CAD build for the part. Positions are in the model's coordinates, mm. A direction names the side the tool comes from. Give positions to 0.01 mm unless a question says otherwise; leave off trailing zeros. Write each loop counter-clockwise with the first axis right and the second up, starting at its lowest first coordinate (ties: lowest second). Pieces come first, ordered by that corner, then holes. Notation, with made-up numbers: M 45.5,62.5 L 50.5,62.5 A27 ccw 50.5,87.5 Z; hole C -9,-27 d5. An arc over 180 degrees is marked long. One line per question, with ' | ' between items. Start each with the question number.
1. Cut at B-B, the plane x = -34. Write the cut outline in (y, z), then the cut area to 4 significant figures.
2. Cut at A-A, the plane y = -2.2. Count the separate pieces of the cut face and the enclosed holes in it, then the cut area to 3 significant figures.
3. Cut at D-D, the plane x = -18. Write the cut outline in (y, z).
4. Pull direction Z, two halves, no side cores. Call faces 1 (the face through (-36.5, 0, -7.5)), 2 (the face through (0, 0, -12)), 3 (the face through (-20.365, 0.036, -0.987)): released by +Z, released by -Z, zero draft, split by the parting line, or undercut.
5. Flat gauge pins, fed straight in: pin 1 (4.5 mm diameter, centred on x = -4.5, z = -3.5, fed in from +Y); pin 2 (2.5 mm diameter, centred on x = -4, z = -3.5, fed in from +Y); pin 3 (0.8 mm diameter, centred on x = -34, z = 0.5, fed in from -Y); pin 4 (0.8 mm diameter, centred on x = -4.5, y = 1.5, fed in from +Z). Where does each tip first touch, or does it go through?
6. Cut at C-C, the plane z = -22.25. Write the cut outline in (x, y).
7. Wall check: L1, parallel to Z at x = -4, y = -1.55; L2, parallel to X at y = -0.65, z = -3.25; L3, parallel to Z at x = -5, y = -2.1. Give the ranges that are in metal, low to high.
8. Which spindle directions (+Z, -Z, +X, -X, +Y, -Y) get a long thin tool onto all of the face, cutting with end or side? Do faces 4 (the face through (-3, 0.1, -23)), 5 (the face through (-17, 0, -2)), 6 (the face through (-9.5, -2.1, 2.5)), 7 (the face through (-36.5, 1.9, -0.5)), 8 (the face through (-36.5, -1.9, -0.5)). Say none if no direction does.
```python
from build123d import *

# Parameters (mm, degrees)
BOSS_EXTRUDE1_DEPTH = 2.6
BOSS_EXTRUDE2_DEPTH = 4
BOSS_EXTRUDE3_DEPTH = 4
SKETCH4_W           = 3
SKETCH4_H           = 5.2
BOSS_EXTRUDE4_DEPTH = 8
BOSS_EXTRUDE5_DEPTH = 2.6
SKETCH6_R           = 1.6
CUT_EXTRUDE1_DEPTH  = 6.2
CUT_EXTRUDE2_DEPTH  = 2.5
CHAMFER1_SIZE       = 1


with BuildPart() as part:
    # Sketch1 → Boss-Extrude1 (new body, symmetric)
    with BuildSketch(Plane(origin=(0, 0, 0), x_dir=(1, 0, 0), z_dir=(0, 1, 0))):
        Polygon((0, 0), (0, 25), (-8, 25), (-8, 8), (-37, 8), (-37, 0), (-33, 0), (-33, 2), (-25, 2), (-25, 0), (-21, 0), (-21, 2), (-13, 2), (-13, 0), align=None)
    extrude(amount=BOSS_EXTRUDE1_DEPTH, both=True)

    # Sketch2 → Boss-Extrude2 (add)
    with BuildSketch(Plane.ZY.offset(13)):
        Polygon((1.5, -1.25), (1.5, -2.6), (4.5, -2.6), (4.5, 2.6), (1.5, 2.6), (1.5, 1.25), (0, 1.25), (0, -1.25), align=None)
    boss_extrude2 = extrude(amount=-BOSS_EXTRUDE2_DEPTH)

    # Sketch3 → Boss-Extrude3 (add)
    with BuildSketch(Plane.ZY.offset(25)):
        Polygon((0, 1.25), (0, -1.25), (1.5, -1.25), (1.5, -2.6), (4.5, -2.6), (4.5, 2.6), (1.5, 2.6), (1.5, 1.25), align=None)
    extrude(amount=-BOSS_EXTRUDE3_DEPTH)

    # Sketch4 → Boss-Extrude4 (add)
    with BuildSketch(Plane.ZY.offset(13)):
        with Locations((3, 0)):
            Rectangle(SKETCH4_W, SKETCH4_H)
    boss_extrude4 = extrude(amount=BOSS_EXTRUDE4_DEPTH)

    # Sketch5 → Boss-Extrude5 (add, symmetric)
    with BuildSketch(Plane(origin=(0, 0, 0), x_dir=(1, 0, 0), z_dir=(0, 1, 0))):
        with BuildLine():
            Line((-13, 1), (-13, 2))
            Line((-13, 2), (-13.535898385, 2))
            ThreePointArc((-13.535898385, 2), (-16.36772326, 0.050287843), (-19.666666667, 1.01857603))
            ThreePointArc((-19.666666667, 1.01857603), (-20.372677996, 0.979231367), (-20.333333333, 0.273220038))
            ThreePointArc((-20.333333333, 0.273220038), (-16.506884, -0.975624243), (-13, 1))
        make_face()
    boss_extrude5 = extrude(amount=BOSS_EXTRUDE5_DEPTH, both=True)

    # Mirror1: Boss-Extrude2, Boss-Extrude4, Boss-Extrude5 across plane
    add(boss_extrude2.mirror(Plane.ZY.offset(23)))
    add(boss_extrude4.mirror(Plane.ZY.offset(23)))
    add(boss_extrude5.mirror(Plane.ZY.offset(23)))

    # Sketch6 → Cut-Extrude1 (cut, through all)
    with BuildSketch(Plane(origin=(0, 2.6, 0), x_dir=(1, 0, 0), z_dir=(0, 1, 0))):
        with Locations((-4, 21.5)):
            Circle(SKETCH6_R)
        with Locations((-4, 3.5)):
            Circle(SKETCH6_R)
    extrude(amount=-CUT_EXTRUDE1_DEPTH, mode=Mode.SUBTRACT)

    # Sketch7 → Cut-Extrude2 (cut)
    with BuildSketch(Plane(origin=(0, 2.6, 0), x_dir=(1, 0, 0), z_dir=(0, 1, 0))):
        Polygon((-0.824573519, 3.5), (-2.41228676, 6.25), (-5.58771324, 6.25), (-7.175426481, 3.5), (-5.58771324, 0.75), (-2.41228676, 0.75), align=None)
        Polygon((-0.824573519, 21.5), (-2.41228676, 24.25), (-5.58771324, 24.25), (-7.175426481, 21.5), (-5.58771324, 18.75), (-2.41228676, 18.75), align=None)
    extrude(amount=-CUT_EXTRUDE2_DEPTH, mode=Mode.SUBTRACT)

    # Chamfer1
    chamfer1_edges = [part.edges().sort_by_distance(p)[0] for p in [
        (-9, 0, 4.5),
        (-9, -2.6, 3),
        (-23, -2.6, 4.5),
        (-9, 2.6, 3),
        (-23, 2.6, 4.5),
        (-37, -2.6, 3),
        (-37, 2.6, 3),
        (-37, 0, 4.5),
        (-37, 1.925, 0),
        (-37, -1.925, 0),
        (-37, 0, -8),
        (-8, 0, -8),
        (0, 0, 0),
        (0, 0, -25),
        (-8, 0, -25),
    ]]
    chamfer(chamfer1_edges, length=CHAMFER1_SIZE)


solid = part.part
```
Here are the results:
1) outline: M -2.6,-8 L 2.6,-8 L 2.6,0 L 1.25,0 L 1.25,1.5 L 2.6,1.5 L 2.6,3.5 L 1.6,4.5 L -1.6,4.5 L -2.6,3.5 L -2.6,1.5 L -1.25,1.5 L -1.25,0 L -2.6,0 Z | area: 59.95 mm^2
2) separate pieces: 2 | enclosed holes: 2 | area: 463 mm^2
3) outline: M -2.6,-8 L 2.6,-8 L 2.6,-2 L -2.6,-2 Z; M -2.6,-0.13 L 2.6,-0.13 L 2.6,0.9 L -2.6,0.9 Z; M -2.6,1.5 L 2.6,1.5 L 2.6,3.5 L 1.6,4.5 L -1.6,4.5 L -2.6,3.5 Z
4) face 1: released by -Z | face 2: zero draft | face 3: undercut
5) pin 1: y = 0.1 | pin 2: through | pin 3: y = -1.25 | pin 4: z = 0
6) outline: M -8,-2.6 L -5.41,-2.6 L -5.41,0.1 L -6.74,0.1 L -6.74,2.6 L -8,2.6 Z; M -2.59,-2.6 L 0,-2.6 L 0,2.6 L -1.26,2.6 L -1.26,0.1 L -2.59,0.1 Z
7) L1: -25 to -23.1, -19.9 to -5.1, -1.9 to 0 | L2: -37 to -5.58, -2.42 to 0 | L3: -25 to -22.75, -20.25 to -4.75, -2.25 to 0
8) face 4: +Y | face 5: +Y, -Y | face 6: +Z, +X, -Y | face 7: -X, +Y | face 8: -X, -Y
